Geometry check sheet. Reference: the model listing, model coordinates, mm. Face numbers are marked on the shaded views. Coordinates: 2 decimals unless noted, no trailing zeros. Write each loop counter-clockwise with the first axis right and the second up, starting at its lowest first coordinate (ties: lowest second). Pieces come first, ordered by that corner, then holes. Notation, with made-up numbers: (-34, 14) -> (10, 14) arc R17 cw to (10, 35) -> close; hole circle Ø6 at (28.5, -19). An arc over 180 degrees is marked (long way). One line per question, with ' | ' between items.
from build123d import *

# Parameters (mm, degrees)
SKETCH2_R               = 26.5
CUT_EXTRUDE1_DEPTH      = 1
CUT_EXTRUDE1_DEPTH_BACK = 71


with BuildPart() as part:
    # Sketch1 → Revolve1 (revolve)
    with BuildSketch(Plane.XY):
        with BuildLine():
            Line((0, 0), (0, 70))
            Line((0, 70), (34.5, 70))
            Line((34.5, 70), (37, 28))
            Line((37, 28), (30, 12.5))
            ThreePointArc((30, 12.5), (31.098349571, 9.848349571), (33.75, 8.75))
            Line((33.75, 8.75), (37, 5.5))
            Line((37, 5.5), (37, 0))
            Line((37, 0), (0, 0))
        make_face()
    revolve(axis=Axis((0, 0, 0), (0, 1, 0)))

    # Sketch2 → Cut-Extrude1 (cut, two sides)
    with BuildSketch(Plane(origin=(0, 70, 0), x_dir=(1, 0, 0), z_dir=(0, 1, 0))) as cut_extrude1_sk:
        Circle(SKETCH2_R)
    extrude(amount=CUT_EXTRUDE1_DEPTH, mode=Mode.SUBTRACT)
    extrude(cut_extrude1_sk.sketch, amount=-CUT_EXTRUDE1_DEPTH_BACK, mode=Mode.SUBTRACT)


solid = part.part
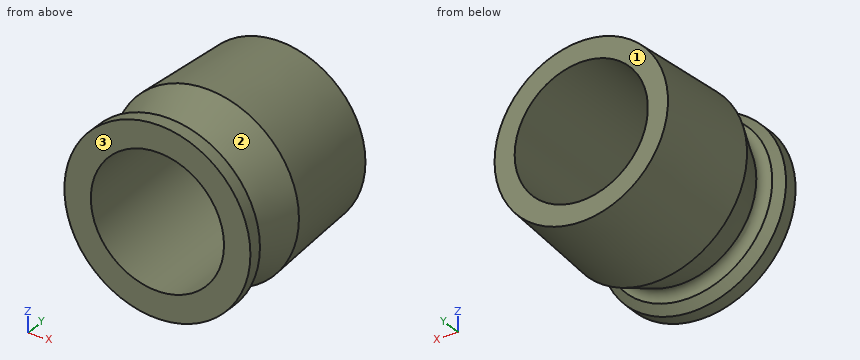
1. Cross-section at C-C on y = 43. Record the boundary of the cut face in (x, z), and give its area (3 significant figures).
Worked answers:
outline: circle Ø72.21 at (0, 0); hole circle Ø53 at (0, 0) | area: 1,890 mm²
2. Cross-section at D-D on y = 58. Record the boundary of the cut face in (x, z), and give its area (3 significant figures).
Worked answers:
outline: circle Ø70.43 at (0, 0); hole circle Ø53 at (0, 0) | area: 1,690 mm²
3. Mould release check, pull along Y, two halves, no side actions. Record for the marked faces 1, 2 and 3: released by +Y, released by -Y, zero draft, split by the parting line, or undercut.
Worked answers:
face 1: released by +Y | face 2: undercut | face 3: released by -Y
4. Material ranges on line 1 (Z direction, x = 6, y = 46); line 2 (Y direction, x = 4, z = 34); line 3 (Z direction, x = -11, y = 39), recorded low to high. Write a range as from..to.
Worked answers:
line 1: -35.42..-25.81, 25.81..35.42 | line 2: 0..8.27, 21.88..70 | line 3: -34.64..-24.11, 24.11..34.64
5. Cross-section at A-A on x = 0. Record the boundary of the cut face in (y, z).
Worked answers:
outline: (0, -37) -> (5.5, -37) -> (8.75, -33.75) arc R3.75 cw to (12.5, -30) -> (28, -37) -> (70, -34.5) -> (70, -26.5) -> (0, -26.5) -> close; (0, 26.5) -> (70, 26.5) -> (70, 34.5) -> (28, 37) -> (12.5, 30) arc R3.75 cw to (8.75, 33.75) -> (5.5, 37) -> (0, 37) -> close
6. Go/stop test with flat-tipped pins: P1, Ø6, axis at x = -9.5, y = 49.5, coming from the -Z side; P2, Ø1, axis at y = 50.5, z = 12, coming from the -X side; P3, Ø3, axis at y = 13, z = -15.5, coming from the -X side. Record where each tip stops, or that it passes through.
Worked answers:
P1: z = -35.15 | P2: x = -33.76 | P3: x = -27.1
7. Cross-section at B-B on z = 0. Record the boundary of the cut face in (x, y), and give its area (3 significant figures).
Worked answers:
outline: (-37, 0) -> (-26.5, 0) -> (-26.5, 70) -> (-34.5, 70) -> (-37, 28) -> (-30, 12.5) arc R3.75 cw to (-33.75, 8.75) -> (-37, 5.5) -> close; (26.5, 0) -> (37, 0) -> (37, 5.5) -> (33.75, 8.75) arc R3.75 cw to (30, 12.5) -> (37, 28) -> (34.5, 70) -> (26.5, 70) -> close | area: 1,200 mm²
